Design review of the part shown in the three views and the two pictorial views. Dimensions are in mm from the part's minimum x, y and z. A direction names the side the tool comes from. Give positions to 0.01 mm unless a question says otherwise; leave off trailing zeros. Loops run counter-clockwise (first coordinate to the right, second up) from the corner with the lowest first, then second, coordinate; pieces in that order, holes last. Notation, with made-up numbers: (-9, 70) -> (7, 70) arc R28 ccw to (7, 94) -> close; hole circle Ø5 at (-40, -21). An arc over 180 degrees is marked (long way). Use CSV: the item, a comma, the result in double quotes. Start each with the question number.
Item 1: We need section C-C (x = 48). State the section outline as (y, z) points.
Item 2: We need section D-D (y = 15.75). State the section outline as (x, z) points, plus the area to 3 significant figures.
Item 3: Clearance check with flat-ended pins moving along their axes: pin 1 (3.5 mm diameter, centred on y = 18.5, z = 10.5, fed in from -X); pin 2 (3 mm diameter, centred on x = 6.5, z = 44.5, fed in from -Y); pin 3 (13 mm diameter, centred on y = 20.5, z = 12, fed in from +X). State where each tip first meets the part, or that it passes through.
Item 4: Wall thickness on line 1 along X through (y, z) = (18.25, 11.5); line 2 along X through (y, z) = (20.75, 34.5) (1 decimal); line 3 along X through (y, z) = (22.5, 32.5): over which ranges is each line inside the solid? List them lowest first. Write a range as from..to.
Item 5: We need section B-B (z = 50). State the section outline as (x, y) points, plus the area to 3 significant figures.
Item 6: For the marked faces 1, 2, 3 and 4, list the 3-axis set-ups (+Z, -Z, +X, -X, +Y, -Y) from which the entire face can be reached by the end or side of a thin tool; tool diameter is ignored.
Item 7: We need section A-A (x = 32.5). State the section outline as (y, z) points, plus the area to 3 significant figures.
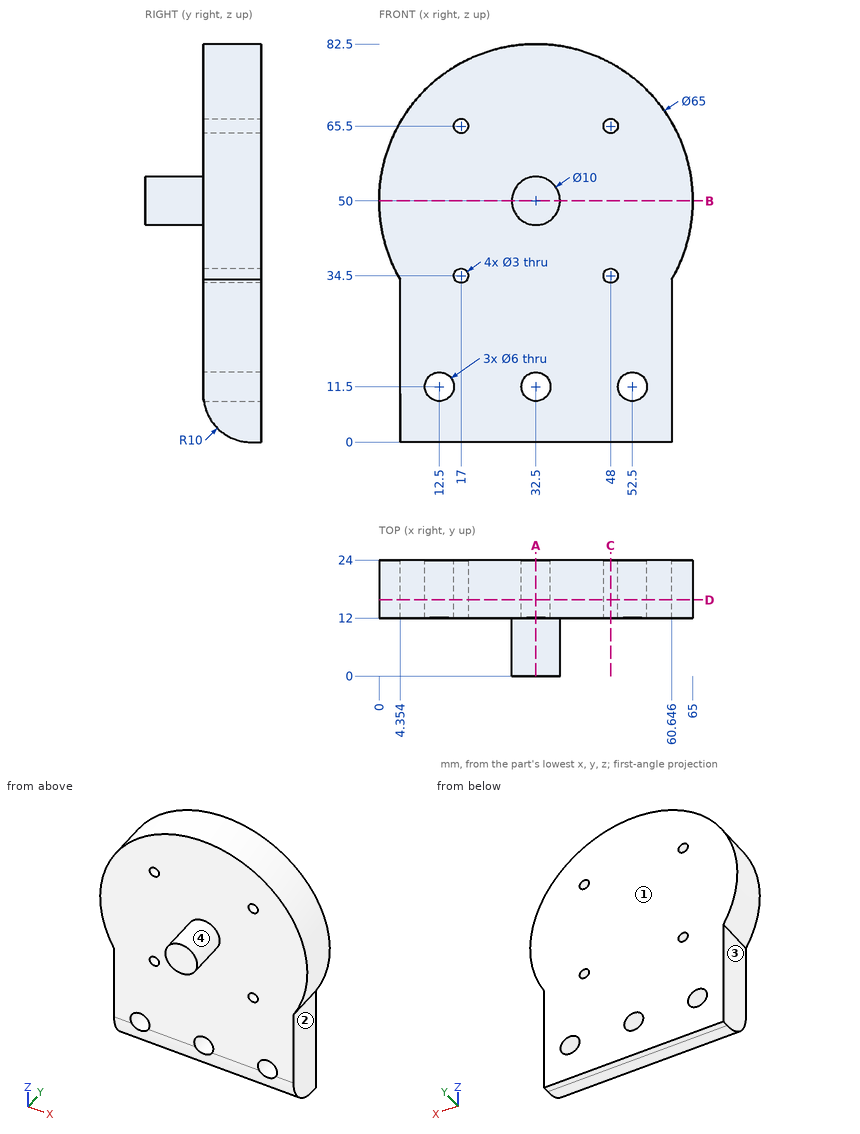
Results found:
1,outline,"(12, 10) arc R10 ccw to (22, 0) -> (24, 0) -> (24, 33) -> (12, 33) -> close; (12, 36) -> (24, 36) -> (24, 64) -> (12, 64) -> close; (12, 67) -> (24, 67) -> (24, 78.57) -> (12, 78.57) -> close"
2,outline,"(4.35, 2.19) -> (60.65, 2.19) -> (60.65, 33.75) arc R32.5 ccw (long way) to (4.35, 33.75) -> close; hole circle Ø6 at (12.5, 11.5); hole circle Ø3 at (17, 34.5); hole circle Ø3 at (17, 65.5); hole circle Ø6 at (32.5, 11.5); hole circle Ø3 at (48, 34.5); hole circle Ø3 at (48, 65.5); hole circle Ø6 at (52.5, 11.5)"
2,area,"4,330 mm²"
3,pin 1,"x = 4.35"
3,pin 2,"y = 12"
3,pin 3,"x = 60.65"
4,line 1,"4.35..9.5, 15.5..29.5, 35.5..49.5, 55.5..60.65"
4,line 2,"3.9..15.5, 18.5..46.5, 49.5..61.1"
4,line 3,"4.35..60.65"
5,outline,"(0, 12) -> (27.5, 12) -> (27.5, 0) -> (37.5, 0) -> (37.5, 12) -> (65, 12) -> (65, 24) -> (0, 24) -> close"
5,area,"900 mm²"
6,face 1,"+Z, -Z, +X, -X, +Y"
6,face 2,"-Z, +X, +Y, -Y"
6,face 3,"-Z, -X, +Y, -Y"
6,face 4,"-Y"
7,outline,"(0, 45) -> (12, 45) -> (12, 14.5) -> (24, 14.5) -> (24, 82.5) -> (12, 82.5) -> (12, 55) -> (0, 55) -> close; (12.11, 8.5) arc R10 ccw to (22, 0) -> (24, 0) -> (24, 8.5) -> close"
7,area,"1,020 mm²"
